```python
from build123d import *

# Parameters (mm, degrees)
F0_W     = 17.4625
F0_H     = 3.175
F2_W     = 13.680584
F2_H     = 12.9563
F3_DEPTH = 0.014764
F4_R     = 3.175
F5_DEPTH = 25.4
F6_SIZE2 = 1.5875
F6_SIZE  = 1.5875


with BuildPart() as f1:
    # F0 (on Right) → F1 (revolve)
    with BuildSketch(Plane.YZ):
        with Locations((-1.412255, 4.7625)):
            Rectangle(F0_W, F0_H)
        Polygon((7.318995, 6.35), (7.318995, 3.175), (47.006495, 3.175), (91.456495, 3.175), (91.456495, 6.35), (73.993995, 6.35), (73.993995, 9.525), (7.318995, 9.525), align=None)
    revolve(axis=Axis((0, 40.656495, 0), (0, 1, 0)))

    # F4 (on face) → F5 (cut)
    with BuildSketch(Plane.YZ.offset(9.525)):
        with Locations((40.656495, 0)):
            Circle(F4_R)
    extrude(amount=-F5_DEPTH, mode=Mode.SUBTRACT)

    # F6
    f6_edges = [f1.edges().sort_by_distance(p)[0] for p in [
        (0, -10.143505, -6.35),
        (0, 91.456495, -6.35),
    ]]
    chamfer(f6_edges, length=F6_SIZE, length2=F6_SIZE2)


with BuildPart() as f3:
    # F2 (on Right) → F3 (new body)
    with BuildSketch(Plane.YZ):
        with Locations((-37.624579, 0)):
            Rectangle(F2_W, F2_H)
    extrude(amount=F3_DEPTH)


solid = f1.part
```
Check sheet for the modelled part. Datum: model origin and axes. Units: mm. A direction names the side the tool comes from. Round coordinates to 2 decimals unless told otherwise and drop trailing zeros. Order: outer loops, then holes, each group sorted by start corner. A loop starts at its lowest first (then second) coordinate and runs counter-clockwise, first axis right, second up.
1) Scan lines: line 1 (X direction, y = 75, z = 0) (3 decimals); line 2 (X direction, y = 28.5, z = 0) (3 decimals); line 3 (Y direction, x = -4, z = -6). Record each from-to range of solid material in increasing order.
2) Section check B-B (y = 34). Record the boundary of the cut face in (x, z) (3 decimals), and give its area (3 significant figures).
3) Section check D-D (y = 5). Record the boundary of the cut face in (x, z) (3 decimals).
4) Section check A-A (z = 0). Give the number of separate pieces and of enclosed holes in the cut face, and give its area (3 significant figures).
5) Mould release check, pull along Z, two halves, no side actions. Record for faces 3 (the cylindrical face through (-6.2, -0.51, -1.38)), 4 (the flat face through (-2, 7.319, 6.2)), 5 (the cylindrical face through (-5.76, 37.485, 0.14)), 6 (the cylindrical face through (5.888, 37.485, 0.14)): +Z half, -Z half, draft (parallel to the pull), parting line (faces both ways), or undercut.
6) Go/stop test with flat-tipped pins: pin 1 Ø5 at (x, z) = (0, 0) entering from -Y; pin 2 Ø1 at (y, z) = (17, 6.5) entering from -X; pin 3 Ø1 at (x, y) = (-6, 78.5) entering from +Z; pin 4 Ø1 at (x, y) = (4, 8) entering from +Z. Record where each tip stops, or that it passes through.
7) Tool access check on faces 1 (the cylindrical face through (-6.2, 81.82, -1.38)), 2 (the cylindrical face through (0.14, 15.61, -3.17)). Record the directions out of +Z, -Z, +X, -X, +Y, -Y that give a thin tool (end or side, any length) a straight path to the whole face; none if there is none.
Result:
1. line 1: x = -6.35 to -3.175, 3.175 to 6.35
1. line 2: x = -9.525 to -3.175, 3.175 to 9.525
1. line 3: y = 7.32 to 73.99
2. outline: circle Ø19.05 at (0, 0); hole circle Ø6.35 at (0, 0)
2. area: 253 mm2
3. outline: circle Ø12.7 at (0, 0); hole circle Ø6.35 at (0, 0)
4. separate pieces: 4
4. enclosed holes: 0
4. area: 983 mm2
5. face 3: parting line
5. face 4: draft
5. face 5: undercut
5. face 6: undercut
6. pin 1: passes through
6. pin 2: stops at x = -7.4
6. pin 3: stops at z = 3.17
6. pin 4: stops at z = 8.86
7. face 1: +Y
7. face 2: +Y, -Y
